```python
from build123d import *

# Parameters (mm, degrees)
EXTRUDE_1_DEPTH     = 165
SKETCH_2_R          = 5
CUT_EXTRUDE_1_DEPTH = 10
SKETCH_3_R          = 5
CUT_EXTRUDE_2_DEPTH = 10
CUT_EXTRUDE_3_DEPTH = 66


with BuildPart() as part:
    # Эскиз1 → Вытянуть-Тонкостенный1 (new body)
    with BuildSketch(Plane(origin=(0, 0, 0), x_dir=(1, 0, 0), z_dir=(0, 1, 0))):
        Polygon((0, 65), (0, 0), (65, 0), (65, 4), (4, 4), (4, 65), align=None)
    extrude(amount=EXTRUDE_1_DEPTH)

    # Эскиз2 → Вырез-Вытянуть1 (cut)
    with BuildSketch(Plane.XY):
        with Locations((31, 145)):
            Circle(SKETCH_2_R)
        with Locations((31, 45)):
            Circle(SKETCH_2_R)
    extrude(amount=-CUT_EXTRUDE_1_DEPTH, mode=Mode.SUBTRACT)

    # Эскиз3 → Вырез-Вытянуть2 (cut)
    with BuildSketch(Plane.ZY):
        with Locations((-31, 145)):
            Circle(SKETCH_3_R)
        with Locations((-31, 45)):
            Circle(SKETCH_3_R)
        with Locations((-15, 10)):
            Circle(SKETCH_3_R)
        with Locations((-45, 10)):
            Circle(SKETCH_3_R)
    extrude(amount=-CUT_EXTRUDE_2_DEPTH, mode=Mode.SUBTRACT)

    # Эскиз4 → Вырез-Вытянуть3 (cut, through all)
    with BuildSketch(Plane.XY):
        Polygon((5, 0), (65, 60), (65, 0), align=None)
    extrude(amount=-CUT_EXTRUDE_3_DEPTH, mode=Mode.SUBTRACT)


solid = part.part
```
Can you work these out from the model? Positions are in its coordinate system, mm. A direction names the side the tool comes from. Coordinates: 2 decimals unless noted, no trailing zeros. Loops run counter-clockwise (first coordinate to the right, second up) from the corner with the lowest first, then second, coordinate; pieces in that order, holes last. Notation, with made-up numbers: (83.25, 82) -> (95.25, 82) arc R23 ccw to (95.25, 93) -> close; hole circle Ø1 at (78.25, 57.5). An arc over 180 degrees is marked (long way). Put each result on its own line as item: value. Start each with the question number.
Q1. I want a section at D-D (z = -31). Write out the boundary of the cut face in (x, y), plus the area to 3 significant figures.
Q2. I want a section at A-A (y = 45). Write out the boundary of the cut face in (x, z).
Q3. I'm going to push flat-ended pins straight in: P1, Ø9, axis at y = 10, z = -45, coming from the +X side; P2, Ø16, axis at y = 45, z = -31, coming from the -X side; P3, Ø13, axis at x = 31, y = 145, coming from the -Z side; P4, Ø1.5, axis at y = 88.5, z = -45.5, coming from the +X side. Where does each tip first touch, or does it pass through?
Q4. If I drill on line 1 (Y direction, x = 31, z = -2.6); line 2 (Y direction, x = 2.05, z = -31); line 3 (Z direction, x = 12.5, y = 59), over which ranges is the centre line in solid material (lowest first)? Write a range as [from, to].
Q5. For faces 4 (the face through (4, 81, -34)), 5 (the face through (32, 100, 0)), which set-ups out of +Z, -Z, +X, -X, +Y, -Y let a thin tool reach every point of the face, with its end or its side?
Q6. I want a section at B-B (x = 31). Write out the boundary of the cut face in (y, z), plus the area to 3 significant figures.
Q7. Thinking about a two-plate mould opening in Y: for faces 1 (the face through (35, 30, -2)), 2 (the face through (2, 13, -19)), 3 (the face through (35, 100, -4)), which applies, pulls with the +Y half, pulls with the -Y half, needs draft (parallel to the pull), parting line crosses it, or undercut?
Q8. I want a section at C-C (z = -45). Write out the boundary of the cut face in (x, y).
Taken from the geometry:
1. outline: (0, 0) -> (4, 0) -> (4, 40) -> (0, 40) -> close; (0, 50) -> (4, 50) -> (4, 140) -> (0, 140) -> close; (0, 150) -> (4, 150) -> (4, 165) -> (0, 165) -> close
1. area: 580 mm2
2. outline: (0, -65) -> (4, -65) -> (4, -36) -> (0, -36) -> close; (0, -26) -> (4, -26) -> (4, -4) -> (26, -4) -> (26, 0) -> (0, 0) -> close; (36, -4) -> (50, -4) -> (50, 0) -> (36, 0) -> close
3. P1: passes through
3. P2: stops at x = 0
3. P3: stops at z = -4
3. P4: stops at x = 4
4. line 1: y = [26, 40], [50, 140], [150, 165]
4. line 2: y = [0, 40], [50, 140], [150, 165]
4. line 3: z = [-4, 0]
5. face 4: -Z, +X, +Y, -Y
5. face 5: +Z, +X, -X, +Y, -Y
6. outline: (26, -4) -> (40, -4) -> (40, 0) -> (26, 0) -> close; (50, -4) -> (140, -4) -> (140, 0) -> (50, 0) -> close; (150, -4) -> (165, -4) -> (165, 0) -> (150, 0) -> close
6. area: 476 mm2
7. face 1: pulls with the -Y half
7. face 2: undercut
7. face 3: needs draft
8. outline: (0, 0) -> (4, 0) -> (4, 5) -> (0, 5) -> close; (0, 15) -> (4, 15) -> (4, 165) -> (0, 165) -> close
